Verification items for the finished model (mm, model axes). A direction names the side the tool comes from. Coordinates: 2 decimals unless noted, no trailing zeros. Order: outer loops, then holes, each group sorted by start corner. A loop starts at its lowest first (then second) coordinate and runs counter-clockwise, first axis right, second up. Notation, with made-up numbers: (44.5, 32.5) -> (57.5, 32.5) arc R14 cw to (57.5, 51.5) -> close; hole circle Ø7 at (13.5, 80.25). An arc over 180 degrees is marked (long way). Write each question's results on one line, items separated by ' | '. Start each with the question number.
(1) Cross-section at A-A on x = -21.1. Enter the section's corners in (y, z).
(2) Draft check along Y on faces 6 (the cylindrical face through (-19.3, 4.05, 3.22)), 7 (the flat face through (-11, -12.5, 3)), 8 (the flat face through (-15, -1, 0)). Enter one of: +Y half, -Y half, draft (parallel to the pull), parting line (faces both ways), or undercut.
(3) Cross-section at D-D on x = -72.1. Enter the section's corners in (y, z), and give its area (3 significant figures).
(4) Set-up check for faces 1 (the flat face through (-75, -2, 3)), 2 (the flat face through (1, 12.5, 3)), 3 (the flat face through (-15, -1, 6.35)), 4 (the flat face through (-47, 10, 3)), 5 (the flat face through (-105, 12, 3)): record each of +Z, -Z, +X, -X, +Y, -Y from which the full face is reachable in a straight line by a thin tool's end or side.
(5) Thickness scan on probe 1 along X at (y, z) = (-1, 6.25); probe 2 along X at (y, z) = (1.5, 2.5); probe 3 along Y at (x, z) = (2.5, 2.5). Record the ranges inside material, lowest first. Write a range as [from, to].
(6) Cross-section at B-B on x = 25. Enter the section's corners in (y, z).
(7) Cross-section at C-C on z = 5.25. Give the number of separate pieces and of enclosed holes in the cut face, and give its area (3 significant figures).
(8) Go/stop test with flat-tipped pins: pin 1 (1.9 mm diameter, centred on x = -45.5, z = 2.5, fed in from +Y); pin 2 (3 mm diameter, centred on y = 4.5, z = 4.5, fed in from -X); pin 3 (4 mm diameter, centred on x = 25, y = 0, fed in from +Z) (3 decimals). Record where each tip stops, or that it passes through.
```python
from build123d import *

# Parameters (mm, degrees)
SKETCH1_W           = 150
SKETCH1_H           = 25
SKETCH1_R           = 2.5
SKETCH1_R_2         = 4.25
BOSS_EXTRUDE1_DEPTH = 6.35
FILLET1_R           = 20
SKETCH2_R           = 1.95
SKETCH2_W           = 40.8
SKETCH2_H           = 20
CUT_EXTRUDE1_DEPTH  = 6.35
SKETCH3_W           = 6.35
SKETCH3_H           = 8
BOSS_EXTRUDE2_DEPTH = 30
FILLET2_R           = 60
FILLET4_R           = 5
FILLET5_R           = 3


with BuildPart() as part:
    # Sketch1 → Boss-Extrude1 (new body)
    with BuildSketch(Plane.XY):
        Rectangle(SKETCH1_W, SKETCH1_H)
        with Locations((65, 0)):
            Circle(SKETCH1_R, mode=Mode.SUBTRACT)
        with Locations((25, 0)):
            Circle(SKETCH1_R, mode=Mode.SUBTRACT)
        with Locations((45, 0)):
            Circle(SKETCH1_R_2, mode=Mode.SUBTRACT)
    extrude(amount=BOSS_EXTRUDE1_DEPTH)

    # Fillet1
    # the kernel refuses this fillet: 20 mm, written as the material it takes off along each edge
    with BuildSketch(Plane(origin=(75, 12.5, -50), x_dir=(-1, 0, 0), z_dir=(0, 0, 1))) as fillet1_piece_1:
        with BuildLine():
            CenterArc((FILLET1_R, FILLET1_R), FILLET1_R, 180, 90)
            Line((0, FILLET1_R), (0, 0))
            Line((0, 0), (FILLET1_R, 0))
        make_face()
    extrude(amount=106.35, mode=Mode.SUBTRACT)
    with BuildSketch(Plane(origin=(75, -12.5, -50), x_dir=(-1, 0, 0), z_dir=(0, 0, 1))) as fillet1_piece_2:
        with BuildLine():
            CenterArc((FILLET1_R, -FILLET1_R), FILLET1_R, 90, 90)
            Line((0, -FILLET1_R), (0, 0))
            Line((0, 0), (FILLET1_R, 0))
        make_face()
    extrude(amount=106.35, mode=Mode.SUBTRACT)

    # Sketch2 → Cut-Extrude1 (cut)
    with BuildSketch(Plane.XY.offset(6.35)):
        with Locations((-72.1, 4.8)):
            Circle(SKETCH2_R)
        with Locations((-72.1, -4.8)):
            Circle(SKETCH2_R)
        with Locations((-21.1, 4.8)):
            Circle(SKETCH2_R)
        with Locations((-21.1, -4.8)):
            Circle(SKETCH2_R)
        with Locations((-46.6, 0)):
            Rectangle(SKETCH2_W, SKETCH2_H)
    extrude(amount=-CUT_EXTRUDE1_DEPTH, mode=Mode.SUBTRACT)

    # Sketch3 → Boss-Extrude2 (add)
    with BuildSketch(Plane.ZY.offset(75)):
        with Locations((3.175, 13.5)):
            Rectangle(SKETCH3_W, SKETCH3_H)
    extrude(amount=BOSS_EXTRUDE2_DEPTH)

    # Fillet2
    # the kernel refuses this fillet: 60 mm, written as the material it adds along each edge
    with BuildSketch(Plane(origin=(-75, 12.5, 0), x_dir=(1, 0, 0), z_dir=(0, 0, 1))) as fillet2_piece_1:
        with BuildLine():
            CenterArc((23.979157617, 60), FILLET2_R, 246.443535691, 23.556464309)
            Line((0, 5), (-0.479583152, 3.9))
            ThreePointArc((-0.479583152, 3.9), (-1.2, 2.5), (-1.2, 0))
            Line((-1.2, 0), (0, -1.2))
            Line((0, -1.2), (23.979157617, -1.2))
            Line((23.979157617, -1.2), (23.979157617, 0))
        make_face()
    extrude(amount=6.35)

    # Fillet4
    fillet4_edges = [part.edges().sort_by_distance(p)[0] for p in [
        (-75, 17.5, 3.175),
    ]]
    fillet(fillet4_edges, radius=FILLET4_R)

    # Fillet5
    fillet5_edges = [part.edges().sort_by_distance(p)[0] for p in [
        (73.540496218, 0, 3.175),
        (-105, 17.5, 3.175),
    ]]
    fillet(fillet5_edges, radius=FILLET5_R)


solid = part.part
```
Results are:
1) outline: (-12.5, 0) -> (-6.75, 0) -> (-6.75, 6.35) -> (-12.5, 6.35) -> close; (-2.85, 0) -> (2.85, 0) -> (2.85, 6.35) -> (-2.85, 6.35) -> close; (6.75, 0) -> (12.5, 0) -> (12.5, 6.35) -> (6.75, 6.35) -> close
2) face 6: undercut | face 7: -Y half | face 8: draft
3) outline: (-12.5, 0) -> (-6.75, 0) -> (-6.75, 6.35) -> (-12.5, 6.35) -> close; (-2.85, 0) -> (2.85, 0) -> (2.85, 6.35) -> (-2.85, 6.35) -> close; (6.75, 0) -> (16.32, 0) -> (16.32, 6.35) -> (6.75, 6.35) -> close | area: 134 mm2
4) face 1: +Z, -Z, -X, -Y | face 2: +Z, -Z, +X, +Y | face 3: +Z, +X, -X, +Y, -Y | face 4: +Z, -Z | face 5: +Z, -Z, -X, +Y, -Y
5) probe 1: x = [-75, -67], [-26.2, 22.71], [27.29, 40.87], [49.13, 62.71], [67.29, 73.08] | probe 2: x = [-75, -67], [-26.2, 23], [27, 41.02], [48.98, 63], [67, 72.86] | probe 3: y = [-12.5, 12.5]
6) outline: (-12.5, 0) -> (-2.5, 0) -> (-2.5, 6.35) -> (-12.5, 6.35) -> close; (2.5, 0) -> (12.5, 0) -> (12.5, 6.35) -> (2.5, 6.35) -> close
7) separate pieces: 1 | enclosed holes: 8 | area: 2,900 mm2
8) pin 1: stops at y = 12.5 | pin 2: stops at x = -75 | pin 3: passes through
